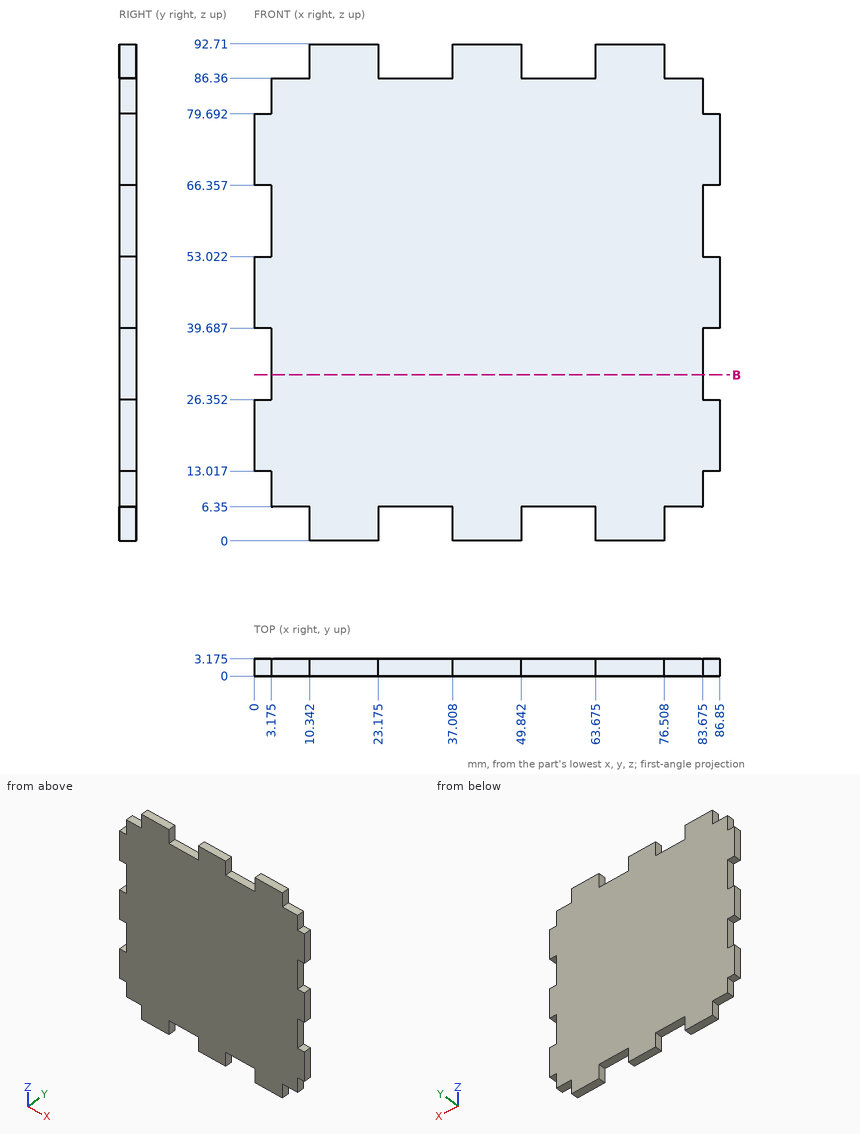
Here's the drawing with two shaded views (mm, measured from the low corner). I have some questions. Round coordinates to 2 decimals unless told otherwise and drop trailing zeros. Loops run counter-clockwise (first coordinate to the right, second up) from the corner with the lowest first, then second, coordinate; pieces in that order, holes last. Notation, with made-up numbers: (16.25, 86.25) - (48.25, 86.25) arc R24 ccw to (48.25, 113.25) - close; hole circle Ø10 at (-29.75, 43). An arc over 180 degrees is marked (long way). Write item = value, one per line.
1) I'm going to push flat-ended pins straight in: P1, Ø1, axis at y = 1.5, z = 90, coming from the +X side; P2, Ø1, axis at y = 2.5, z = 84, coming from the +X side (1 decimal); P3, Ø1, axis at x = 32, y = 2.5, coming from the +Z side. Where does each tip first touch, or does it pass through?
Computed:
P1 = 76.51
P2 = 83.7
P3 = 86.36
2) I need wall thicknesses on line 1 along X through (y, z) = (0.4, 88) (1 decimal); line 2 along Z through (x, y) = (83, 1.95); line 3 along X through (y, z) = (1, 8) (1 decimal). Which ranges of each line are inside material? Lowest first, please. Write a range as from..to.
Computed:
line_1 = 10.3..23.2, 37..49.8, 63.7..76.5
line_2 = 6.35..86.36
line_3 = 3.2..83.7
3) Imagine slicing it at B-B (z = 31). Please give me the cut outline in (x, y) (1 decimal).
Computed:
outline = (3.2, 0) - (83.7, 0) - (83.7, 3.2) - (3.2, 3.2) - close
